The model under review builds one solid part; all positions refer to its coordinate system, in mm. Give positions to 0.01 mm unless a question says otherwise; leave off trailing zeros. Loops run counter-clockwise (first coordinate to the right, second up) from the corner with the lowest first, then second, coordinate; pieces in that order, holes last. Notation, with made-up numbers: M -22.5,27.25 L -12.5,27.25 A25 cw -12.5,48.25 Z; hole C -25.75,58 d1. An arc over 180 degrees is marked long. Return JSON: item names as keys, results as strings.
```python
from build123d import *

# Parameters (mm, degrees)
F0_R     = 1.5875
F1_DEPTH = 30.0736
F2_SIZE  = 0.254
F6_R     = 0.508
F7_DEPTH = 5.59535


with BuildPart() as f1:
    # F0 (on Front) → F1 (new body)
    with BuildSketch(Plane.XZ):
        Circle(F0_R)
    extrude(amount=F1_DEPTH)

    # F2
    f2_edges = [f1.edges().sort_by_distance(p)[0] for p in [
        (-1.5875, 0, 0),
    ]]
    chamfer(f2_edges, length=F2_SIZE)

    # F4: sweep along a path in F4_path
    with BuildLine(Plane(origin=(1.5875, -30.0736, 0), x_dir=(0, 0, -1), z_dir=(0, 1, 0))) as f4_path:
        CenterArc((0, 1.5875), 1.5875, 0, 360)
    # F3 (on Right) → F4 (sweep)
    with BuildSketch(Plane.YZ):
        Polygon((-30.0736, 0), (-30.0736, 1.5875), (-32.3596, 3.96875), (-32.766, 3.96875), (-32.766, 0), align=None)
    sweep(path=f4_path.line)

    # F6 (on offset) → F7 (cut, through all)
    with BuildSketch(Plane.YZ.offset(1.6256)):
        with Locations((-1.6002, 0)):
            Circle(F6_R)
    extrude(amount=-F7_DEPTH, mode=Mode.SUBTRACT)


solid = f1.part
```
1) Wall thickness on L1, parallel to Y at x = -0.1, z = 0; L2, parallel to Z at x = 0, y = -2; L3, parallel to X at y = -18, z = 1.25: over which ranges is each line inside the solid? List them lowest first. Write a range as from..to.
From the geometry:
{"L1": "-32.77..-2.11, -1.09..0", "L2": "-1.59..-0.31, 0.31..1.59", "L3": "-0.98..0.98"}
2) Insertion check: pin 1 (2 mm diameter, centred on x = 2.5, z = -2.5, fed in from +Y); pin 2 (0.8 mm diameter, centred on y = -1.6, z = 0, fed in from +X); pin 3 (1 mm diameter, centred on x = 1.5, y = -4, fed in from +Z). Each pin has a flat end and moves straight along its axis. Give the tip position at first contact, or say it passes through.
From the geometry:
{"pin 1": "y = -30.98", "pin 2": "through", "pin 3": "z = 1.23"}
3) The part is to be moulded in two halves that separate along Y. For faces 1 (the face through (0.022, -1.116, 0.153)), 2 (the face through (3.874, -32.566, 0.86)), 3 (the face through (0, 0, 0)), say which applies: released by +Y, released by -Y, zero draft, split by the parting line, or undercut.
From the geometry:
{"face 1": "undercut", "face 2": "zero draft", "face 3": "released by +Y"}
4) Consider section A-A on y = -4.5. Write out the cut boundary in (x, z) (1 decimal), then the cut area to 3 significant figures.
From the geometry:
{"outline": "C 0,0 d3.2", "area": "7.92 mm²"}
